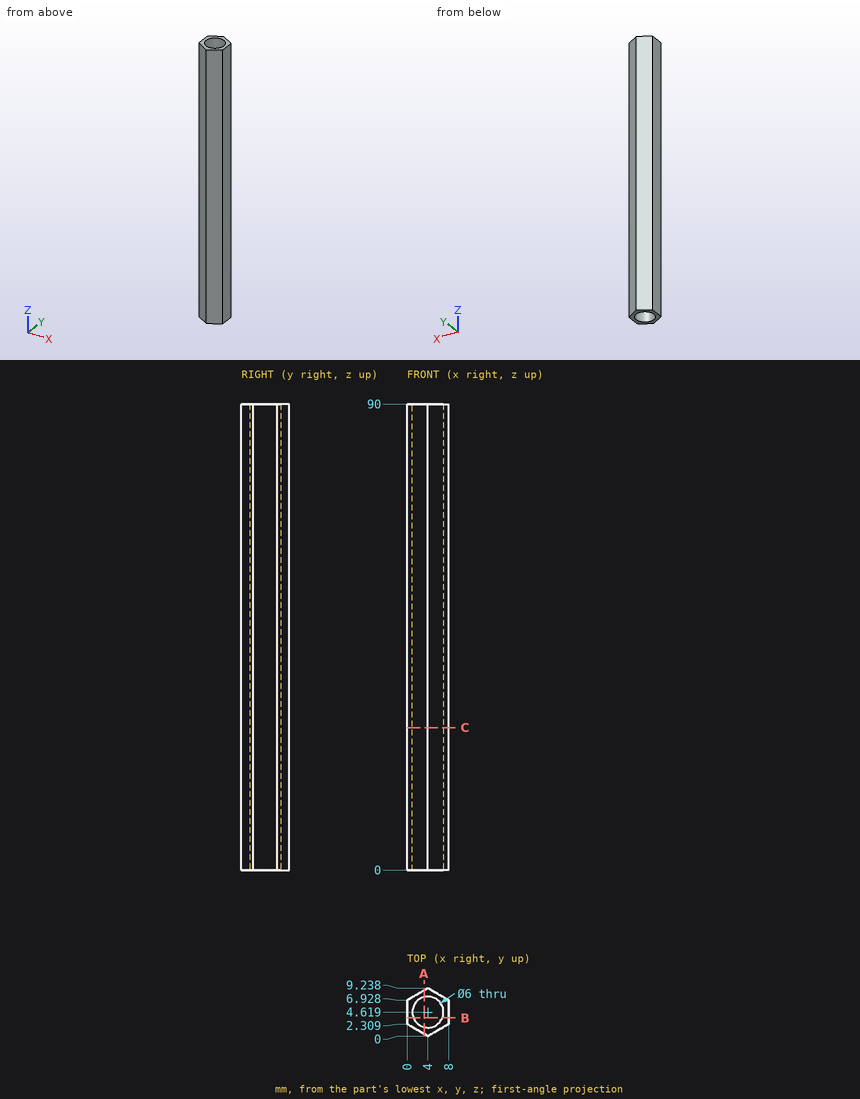
Geometry check sheet. Reference: drawing and pictorial views, mm from the part's lowest x, y, z. Round coordinates to 2 decimals unless told otherwise and drop trailing zeros. Loops run counter-clockwise (first coordinate to the right, second up) from the corner with the lowest first, then second, coordinate; pieces in that order, holes last. Notation, with made-up numbers: (19.25, 23.5) - (41.25, 23.5) arc R19 cw to (41.25, 30.5) - close; hole circle Ø6 at (76, 88). An arc over 180 degrees is marked (long way). Use a Markdown table: item, result. Add a question column.
1. Section check C-C, the plane z = 27.5. Record the boundary of the cut face in (x, y).
2. Section check B-B, the plane y = 3.5. Record the boundary of the cut face in (x, z), plus the area to 3 significant figures.
3. Section check A-A, the plane x = 3.25. Record the boundary of the cut face in (y, z) (1 decimal).
4. Thickness scan on probe 1 along Y at (x, z) = (4, 56.5); probe 2 along X at (y, z) = (5, 17) (1 decimal); probe 3 along Y at (x, z) = (2.75, 79) (1 decimal). Record the ranges inside material, lowest first. Write a range as [from, to].
5. Gauge pin test, flat ends, axial feed: pin 1 (2 mm diameter, centred on y = 1.5, z = 14.5, fed in from -X); pin 2 (1 mm diameter, centred on x = 2.5, z = 80, fed in from -Y). Record the tip position at first contact, or that the pin passes through.
Checks:
| question | item | result |
|---|---|---|
| 1 | outline | (0, 2.31) - (4, 0) - (8, 2.31) - (8, 6.93) - (4, 9.24) - (0, 6.93) - close; hole circle Ø6 at (4, 4.62) |
| 2 | outline | (0, 0) - (1.22, 0) - (1.22, 90) - (0, 90) - close; (6.78, 0) - (8, 0) - (8, 90) - (6.78, 90) - close |
| 2 | area | 219 mm^2 |
| 3 | outline | (0.4, 0) - (1.7, 0) - (1.7, 90) - (0.4, 90) - close; (7.5, 0) - (8.8, 0) - (8.8, 90) - (7.5, 90) - close |
| 4 | probe 1 | y = [0, 1.62], [7.62, 9.24] |
| 4 | probe 2 | x = [0, 1], [7, 8] |
| 4 | probe 3 | y = [0.7, 1.9], [7.3, 8.5] |
| 5 | pin 1 | stops at x = 0 |
| 5 | pin 2 | stops at y = 0.58 |
